from build123d import *

# Parameters (mm, degrees)
BOX009_W     = 1
BOX009_H     = 1
BOX009_DEPTH = 1
BOX008_W     = 1
BOX008_H     = 1
BOX008_DEPTH = 1
BOX007_W     = 1
BOX007_H     = 1
BOX007_DEPTH = 1
BOX006_W     = 1
BOX006_H     = 1
BOX006_DEPTH = 1
BOX005_W     = 1
BOX005_H     = 1
BOX005_DEPTH = 1
BOX003_W     = 3
BOX003_H     = 3
BOX003_DEPTH = 6
BOX015_W     = 1
BOX015_H     = 1
BOX015_DEPTH = 1
BOX014_W     = 1
BOX014_H     = 1
BOX014_DEPTH = 1
BOX013_W     = 1
BOX013_H     = 1
BOX013_DEPTH = 1
BOX012_W     = 1
BOX012_H     = 1
BOX012_DEPTH = 1
BOX011_W     = 1
BOX011_H     = 1
BOX011_DEPTH = 1
BOX010_W     = 3
BOX010_H     = 3
BOX010_DEPTH = 6
BOX021_W     = 1
BOX021_H     = 1
BOX021_DEPTH = 1
BOX020_W     = 1
BOX020_H     = 1
BOX020_DEPTH = 1
BOX019_W     = 1
BOX019_H     = 1
BOX019_DEPTH = 1
BOX018_W     = 1
BOX018_H     = 1
BOX018_DEPTH = 1
BOX017_W     = 1
BOX017_H     = 1
BOX017_DEPTH = 1
BOX016_W     = 3
BOX016_H     = 3
BOX016_DEPTH = 6
BOX027_W     = 1
BOX027_H     = 1
BOX027_DEPTH = 1
BOX026_W     = 1
BOX026_H     = 1
BOX026_DEPTH = 1
BOX025_W     = 1
BOX025_H     = 1
BOX025_DEPTH = 1
BOX024_W     = 1
BOX024_H     = 1
BOX024_DEPTH = 1
BOX023_W     = 1
BOX023_H     = 1
BOX023_DEPTH = 1
BOX022_W     = 3
BOX022_H     = 3
BOX022_DEPTH = 6
BOX002_W     = 2
BOX002_H     = 10
BOX002_DEPTH = 2.5
BOX001_W     = 8
BOX001_H     = 8
BOX001_DEPTH = 10
BOX_W        = 10
BOX_H        = 10
BOX_DEPTH    = 3.5


with BuildPart() as cubo009:
    # Box009 → Box009 (new body)
    with BuildSketch(Plane(origin=(-2, 1, 5), x_dir=(1, 0, 0), z_dir=(0, 0, 1))):
        with Locations((0.5, 0.5)):
            Rectangle(BOX009_W, BOX009_H)
    extrude(amount=BOX009_DEPTH)


with BuildPart() as cubo008:
    # Box008 → Box008 (new body)
    with BuildSketch(Plane(origin=(-4, 1, 5), x_dir=(1, 0, 0), z_dir=(0, 0, 1))):
        with Locations((0.5, 0.5)):
            Rectangle(BOX008_W, BOX008_H)
    extrude(amount=BOX008_DEPTH)


with BuildPart() as cubo007:
    # Box007 → Box007 (new body)
    with BuildSketch(Plane(origin=(-3, 1, 5), x_dir=(1, 0, 0), z_dir=(0, 0, 1))):
        with Locations((0.5, 0.5)):
            Rectangle(BOX007_W, BOX007_H)
    extrude(amount=BOX007_DEPTH)


with BuildPart() as cubo006:
    # Box006 → Box006 (new body)
    with BuildSketch(Plane(origin=(-3, 2, 5), x_dir=(1, 0, 0), z_dir=(0, 0, 1))):
        with Locations((0.5, 0.5)):
            Rectangle(BOX006_W, BOX006_H)
    extrude(amount=BOX006_DEPTH)


with BuildPart() as cubo005:
    # Box005 → Box005 (new body)
    with BuildSketch(Plane(origin=(-3, 0, 5), x_dir=(1, 0, 0), z_dir=(0, 0, 1))):
        with Locations((0.5, 0.5)):
            Rectangle(BOX005_W, BOX005_H)
    extrude(amount=BOX005_DEPTH)


with BuildPart() as cut006:
    # Box003 → Box003 (new body)
    with BuildSketch(Plane(origin=(-4, 0, 0), x_dir=(1, 0, 0), z_dir=(0, 0, 1))):
        with Locations((1.5, 1.5)):
            Rectangle(BOX003_W, BOX003_H)
    extrude(amount=BOX003_DEPTH)

    # Cut002: cut Cubo005
    add(cubo005.part, mode=Mode.SUBTRACT)

    # Cut003: cut Cubo006
    add(cubo006.part, mode=Mode.SUBTRACT)

    # Cut004: cut Cubo007
    add(cubo007.part, mode=Mode.SUBTRACT)

    # Cut005: cut Cubo008
    add(cubo008.part, mode=Mode.SUBTRACT)

    # Cut006: cut Cubo009
    add(cubo009.part, mode=Mode.SUBTRACT)


with BuildPart() as cut006_1:
    # Cut006 placement: moved
    add(cut006.part.moved(Location((12, -1, 0))))


with BuildPart() as cubo015:
    # Box015 → Box015 (new body)
    with BuildSketch(Plane(origin=(-2, 1, 5), x_dir=(1, 0, 0), z_dir=(0, 0, 1))):
        with Locations((0.5, 0.5)):
            Rectangle(BOX015_W, BOX015_H)
    extrude(amount=BOX015_DEPTH)


with BuildPart() as cubo014:
    # Box014 → Box014 (new body)
    with BuildSketch(Plane(origin=(-4, 1, 5), x_dir=(1, 0, 0), z_dir=(0, 0, 1))):
        with Locations((0.5, 0.5)):
            Rectangle(BOX014_W, BOX014_H)
    extrude(amount=BOX014_DEPTH)


with BuildPart() as cubo013:
    # Box013 → Box013 (new body)
    with BuildSketch(Plane(origin=(-3, 1, 5), x_dir=(1, 0, 0), z_dir=(0, 0, 1))):
        with Locations((0.5, 0.5)):
            Rectangle(BOX013_W, BOX013_H)
    extrude(amount=BOX013_DEPTH)


with BuildPart() as cubo012:
    # Box012 → Box012 (new body)
    with BuildSketch(Plane(origin=(-3, 2, 5), x_dir=(1, 0, 0), z_dir=(0, 0, 1))):
        with Locations((0.5, 0.5)):
            Rectangle(BOX012_W, BOX012_H)
    extrude(amount=BOX012_DEPTH)


with BuildPart() as cubo011:
    # Box011 → Box011 (new body)
    with BuildSketch(Plane(origin=(-3, 0, 5), x_dir=(1, 0, 0), z_dir=(0, 0, 1))):
        with Locations((0.5, 0.5)):
            Rectangle(BOX011_W, BOX011_H)
    extrude(amount=BOX011_DEPTH)


with BuildPart() as cut011:
    # Box010 → Box010 (new body)
    with BuildSketch(Plane(origin=(-4, 0, 0), x_dir=(1, 0, 0), z_dir=(0, 0, 1))):
        with Locations((1.5, 1.5)):
            Rectangle(BOX010_W, BOX010_H)
    extrude(amount=BOX010_DEPTH)

    # Cut007: cut Cubo011
    add(cubo011.part, mode=Mode.SUBTRACT)

    # Cut008: cut Cubo012
    add(cubo012.part, mode=Mode.SUBTRACT)

    # Cut009: cut Cubo013
    add(cubo013.part, mode=Mode.SUBTRACT)

    # Cut010: cut Cubo014
    add(cubo014.part, mode=Mode.SUBTRACT)

    # Cut011: cut Cubo015
    add(cubo015.part, mode=Mode.SUBTRACT)


with BuildPart() as cut011_1:
    # Cut011 placement: moved
    add(cut011.part.moved(Location((3, -1, 0))))


with BuildPart() as cubo021:
    # Box021 → Box021 (new body)
    with BuildSketch(Plane(origin=(-2, 1, 5), x_dir=(1, 0, 0), z_dir=(0, 0, 1))):
        with Locations((0.5, 0.5)):
            Rectangle(BOX021_W, BOX021_H)
    extrude(amount=BOX021_DEPTH)


with BuildPart() as cubo020:
    # Box020 → Box020 (new body)
    with BuildSketch(Plane(origin=(-4, 1, 5), x_dir=(1, 0, 0), z_dir=(0, 0, 1))):
        with Locations((0.5, 0.5)):
            Rectangle(BOX020_W, BOX020_H)
    extrude(amount=BOX020_DEPTH)


with BuildPart() as cubo019:
    # Box019 → Box019 (new body)
    with BuildSketch(Plane(origin=(-3, 1, 5), x_dir=(1, 0, 0), z_dir=(0, 0, 1))):
        with Locations((0.5, 0.5)):
            Rectangle(BOX019_W, BOX019_H)
    extrude(amount=BOX019_DEPTH)


with BuildPart() as cubo018:
    # Box018 → Box018 (new body)
    with BuildSketch(Plane(origin=(-3, 2, 5), x_dir=(1, 0, 0), z_dir=(0, 0, 1))):
        with Locations((0.5, 0.5)):
            Rectangle(BOX018_W, BOX018_H)
    extrude(amount=BOX018_DEPTH)


with BuildPart() as cubo017:
    # Box017 → Box017 (new body)
    with BuildSketch(Plane(origin=(-3, 0, 5), x_dir=(1, 0, 0), z_dir=(0, 0, 1))):
        with Locations((0.5, 0.5)):
            Rectangle(BOX017_W, BOX017_H)
    extrude(amount=BOX017_DEPTH)


with BuildPart() as cut016:
    # Box016 → Box016 (new body)
    with BuildSketch(Plane(origin=(-4, 0, 0), x_dir=(1, 0, 0), z_dir=(0, 0, 1))):
        with Locations((1.5, 1.5)):
            Rectangle(BOX016_W, BOX016_H)
    extrude(amount=BOX016_DEPTH)

    # Cut012: cut Cubo017
    add(cubo017.part, mode=Mode.SUBTRACT)

    # Cut013: cut Cubo018
    add(cubo018.part, mode=Mode.SUBTRACT)

    # Cut014: cut Cubo019
    add(cubo019.part, mode=Mode.SUBTRACT)

    # Cut015: cut Cubo020
    add(cubo020.part, mode=Mode.SUBTRACT)

    # Cut016: cut Cubo021
    add(cubo021.part, mode=Mode.SUBTRACT)


with BuildPart() as cut016_1:
    # Cut016 placement: moved
    add(cut016.part.moved(Location((3, 8, 0))))


with BuildPart() as cubo027:
    # Box027 → Box027 (new body)
    with BuildSketch(Plane(origin=(-2, 1, 5), x_dir=(1, 0, 0), z_dir=(0, 0, 1))):
        with Locations((0.5, 0.5)):
            Rectangle(BOX027_W, BOX027_H)
    extrude(amount=BOX027_DEPTH)


with BuildPart() as cubo026:
    # Box026 → Box026 (new body)
    with BuildSketch(Plane(origin=(-4, 1, 5), x_dir=(1, 0, 0), z_dir=(0, 0, 1))):
        with Locations((0.5, 0.5)):
            Rectangle(BOX026_W, BOX026_H)
    extrude(amount=BOX026_DEPTH)


with BuildPart() as cubo025:
    # Box025 → Box025 (new body)
    with BuildSketch(Plane(origin=(-3, 1, 5), x_dir=(1, 0, 0), z_dir=(0, 0, 1))):
        with Locations((0.5, 0.5)):
            Rectangle(BOX025_W, BOX025_H)
    extrude(amount=BOX025_DEPTH)


with BuildPart() as cubo024:
    # Box024 → Box024 (new body)
    with BuildSketch(Plane(origin=(-3, 2, 5), x_dir=(1, 0, 0), z_dir=(0, 0, 1))):
        with Locations((0.5, 0.5)):
            Rectangle(BOX024_W, BOX024_H)
    extrude(amount=BOX024_DEPTH)


with BuildPart() as cubo023:
    # Box023 → Box023 (new body)
    with BuildSketch(Plane(origin=(-3, 0, 5), x_dir=(1, 0, 0), z_dir=(0, 0, 1))):
        with Locations((0.5, 0.5)):
            Rectangle(BOX023_W, BOX023_H)
    extrude(amount=BOX023_DEPTH)


with BuildPart() as cut021:
    # Box022 → Box022 (new body)
    with BuildSketch(Plane(origin=(-4, 0, 0), x_dir=(1, 0, 0), z_dir=(0, 0, 1))):
        with Locations((1.5, 1.5)):
            Rectangle(BOX022_W, BOX022_H)
    extrude(amount=BOX022_DEPTH)

    # Cut017: cut Cubo023
    add(cubo023.part, mode=Mode.SUBTRACT)

    # Cut018: cut Cubo024
    add(cubo024.part, mode=Mode.SUBTRACT)

    # Cut019: cut Cubo025
    add(cubo025.part, mode=Mode.SUBTRACT)

    # Cut020: cut Cubo026
    add(cubo026.part, mode=Mode.SUBTRACT)

    # Cut021: cut Cubo027
    add(cubo027.part, mode=Mode.SUBTRACT)


with BuildPart() as cut021_1:
    # Cut021 placement: moved
    add(cut021.part.moved(Location((12, 8, 0))))


with BuildPart() as cubo002:
    # Box002 → Box002 (new body)
    with BuildSketch(Plane(origin=(4, -3, 0), x_dir=(1, 0, 0), z_dir=(0, 0, 1))):
        with Locations((1, 5)):
            Rectangle(BOX002_W, BOX002_H)
    extrude(amount=BOX002_DEPTH)


with BuildPart() as cubo001:
    # Box001 → Box001 (new body)
    with BuildSketch(Plane(origin=(1, 1, -2), x_dir=(1, 0, 0), z_dir=(0, 0, 1))):
        with Locations((4, 4)):
            Rectangle(BOX001_W, BOX001_H)
    extrude(amount=BOX001_DEPTH)


with BuildPart() as fusion:
    # Box → Box (new body)
    with BuildSketch(Plane.XY):
        with Locations((5, 5)):
            Rectangle(BOX_W, BOX_H)
    extrude(amount=BOX_DEPTH)

    # Cut: cut Cubo001
    add(cubo001.part, mode=Mode.SUBTRACT)

    # Cut001: cut Cubo002
    add(cubo002.part, mode=Mode.SUBTRACT)

    # Fusion: union Cut006, Cut011, Cut016, Cut021
    add(cut006_1.part)
    add(cut011_1.part)
    add(cut016_1.part)
    add(cut021_1.part)


solid = fusion.part
Work out the finished part from the listing and answer in its coordinate system (mm). A direction names the side the tool comes from. Give positions to 0.01 mm unless a question says otherwise; leave off trailing zeros. Order: outer loops, then holes, each group sorted by start corner. A loop starts at its lowest first (then second) coordinate and runs counter-clockwise, first axis right, second up. Notation, with made-up numbers: (35.25, 15) -> (65.25, 15) arc R28 cw to (65.25, 35) -> close; hole circle Ø9 at (32, 55.5). An arc over 180 degrees is marked (long way). One line per item, written item: value.
Item 1: Find section B-B, the plane x = 5. Give the vertices of the cut face in (y, z), plus the area to 3 significant figures.
Answer sheet:
outline: (0, 2.5) -> (1, 2.5) -> (1, 3.5) -> (0, 3.5) -> close; (9, 0) -> (10, 0) -> (10, 3.5) -> (9, 3.5) -> close
area: 4.50 mm²
Item 2: Find section C-C, the plane z = 4.1. Give the vertices of the cut face in (x, y), plus the area to 3 significant figures.
Answer sheet:
outline: (-1, -1) -> (2, -1) -> (2, 2) -> (-1, 2) -> close; (-1, 8) -> (2, 8) -> (2, 11) -> (-1, 11) -> close; (8, -1) -> (11, -1) -> (11, 2) -> (8, 2) -> close; (8, 8) -> (11, 8) -> (11, 11) -> (8, 11) -> close
area: 36.0 mm²
Item 3: A tool of negligible diameter and unlimited length cuts with its end or side. For faces 4 (the flat face through (8, 0, 4)), 5 (the flat face through (1.5, 10, 5.5)), 6 (the flat face through (10, -0.5, 5.5)), 7 (the flat face through (5, 9, 2)), from which of +Z, -Z, +X, -X, +Y, -Y can it reach the whole face along a straight path? Write none if from no direction.
Answer sheet:
face 4: +Z
face 5: +Z, +X, -X
face 6: +Z, +Y, -Y
face 7: +Z, -Z
Item 4: Determine the mould class of faces 1 (the flat face through (10.5, 8.5, 6)), 2 (the flat face through (10, 5, 2)), 3 (the flat face through (9.5, 9.5, 5)) for opening direction X: released by +X, released by -X, zero draft, split by the parting line, or undercut.
Answer sheet:
face 1: zero draft
face 2: released by +X
face 3: undercut
Item 5: Find section D-D, the plane x = 9.5. Give the vertices of the cut face in (y, z), plus the area to 3 significant figures.
Answer sheet:
outline: (-1, 0) -> (11, 0) -> (11, 5) -> (8, 5) -> (8, 3.5) -> (2, 3.5) -> (2, 5) -> (-1, 5) -> close
area: 51.0 mm²
Item 6: Straight lines are drawn through the part: probe 1 along X at (y, z) = (9, 3.9); probe 2 along Y at (x, z) = (3.5, 2.8). For each, find the intervals that lie inside material, in ascending order.
Answer sheet:
probe 1: -1 to 2, 8 to 11
probe 2: 0 to 1, 9 to 10
Item 7: Find section A-A, the plane y = 7. Give the vertices of the cut face in (x, z), plus the area to 3 significant figures.
Answer sheet:
outline: (0, 0) -> (1, 0) -> (1, 3.5) -> (0, 3.5) -> close; (9, 0) -> (10, 0) -> (10, 3.5) -> (9, 3.5) -> close
area: 7.00 mm²
Item 8: Flat-ended cylindrical pins translate along their axes: P1, Ø3, axis at x = 4, z = 3.5, coming from the -Y side; P2, Ø0.5, axis at x = 6, y = 9.5, coming from the +Z side. Find the tip coordinate at first contact, or state that the pin passes through.
Answer sheet:
P1: y = 0
P2: z = 3.5
